For this review, use the dimensioned drawing (mm, ordinates from the lowest corner) and the shaded views. Round coordinates to 2 decimals unless told otherwise and drop trailing zeros. Loops run counter-clockwise (first coordinate to the right, second up) from the corner with the lowest first, then second, coordinate; pieces in that order, holes last. Notation, with made-up numbers: (77, 58) -> (103, 58) arc R22 ccw to (103, 81) -> close; hole circle Ø10 at (-9, 37.5). An arc over 180 degrees is marked (long way). Use one line per item in the form item = value. Start each with the question number.
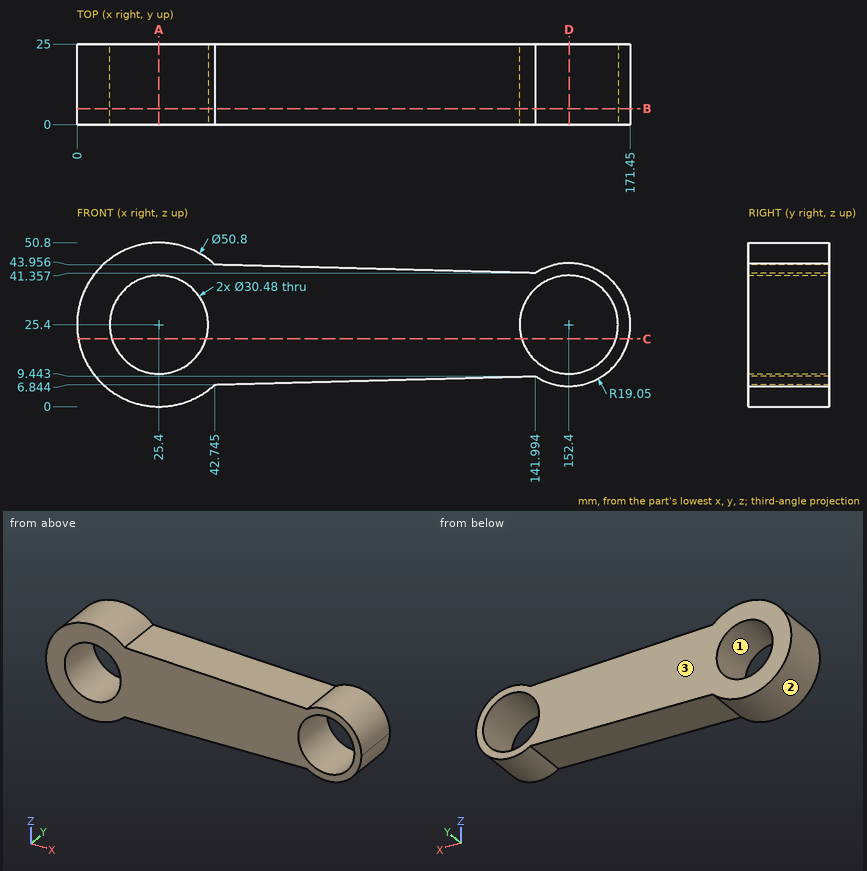
Item 1: Wall thickness on line 1 (X direction, y = 6.5, z = 25.4); line 2 (X direction, y = 3.5, z = 31) (1 decimal); line 3 (Z direction, x = 152.4, y = 10.25): over which ranges is each line inside the solid? List them lowest first.
Item 2: Take a section at C-C on z = 21. Give the boundary of the cut face in (x, y) (1 decimal).
Item 3: Draft analysis for pull direction Z (two halves, no side actions). For the marked faces 1, 2 and 3, state which applies: +Z half, -Z half, draft (parallel to the pull), parting line (faces both ways), or undercut.
Item 4: Take a section at D-D on x = 152.5. Give the boundary of the cut face in (y, z).
Item 5: Take a section at A-A on x = 25.4. Give the boundary of the cut face in (y, z), plus the area to 3 significant figures.
Item 6: Take a section at B-B on y = 5. Give the number of separate pieces and of enclosed holes in the cut face, plus the area to 3 significant figures.
Item 7: For P1, Ø18.5, axis at x = 152.4, z = 25.4, coming from the +Y side; P2, Ø6, axis at x = 33, y = 8, coming from the +Z side; P3, Ø2, axis at x = 23.5, y = 13.5, coming from the +Z side; P4, Ø6, axis at y = 17, z = 32, coming from the -X side, all flat-tipped, find the tip position at first contact; note any pin that passes through.
Results:
q1.line_1 = 0 to 10.16, 40.64 to 137.16, 167.64 to 171.45
q1.line_2 = 0.6 to 11.2, 39.6 to 138.2, 166.6 to 170.6
q1.line_3 = 6.35 to 10.16, 40.64 to 44.45
q2.outline = (0.4, 0) -> (10.8, 0) -> (10.8, 25) -> (0.4, 25) -> close; (40, 0) -> (137.8, 0) -> (137.8, 25) -> (40, 25) -> close; (167, 0) -> (170.9, 0) -> (170.9, 25) -> (167, 25) -> close
q3.face_1 = undercut
q3.face_2 = parting line
q3.face_3 = draft
q4.outline = (0, 6.35) -> (25, 6.35) -> (25, 10.16) -> (0, 10.16) -> close; (0, 40.64) -> (25, 40.64) -> (25, 44.45) -> (0, 44.45) -> close
q5.outline = (0, 0) -> (25, 0) -> (25, 10.16) -> (0, 10.16) -> close; (0, 40.64) -> (25, 40.64) -> (25, 50.8) -> (0, 50.8) -> close
q5.area = 508 mm2
q6.separate_pieces = 1
q6.enclosed_holes = 2
q6.area = 4,730 mm2
q7.P1 = through
q7.P2 = 50.38
q7.P3 = 50.78
q7.P4 = 0.26
